Geometry: see drawing. Coordinates: mm, zero at the bounding-box minimum. A direction names the side the tool comes from. Round coordinates to 2 decimals unless told otherwise and drop trailing zeros. Order: outer loops, then holes, each group sorted by start corner. A loop starts at its lowest first (then second) coordinate and runs counter-clockwise, first axis right, second up. Notation, with made-up numbers: (58.25, 85.5) -> (112.25, 85.5) arc R19 cw to (112.25, 101.5) -> close; hole circle Ø1 at (69, -15.75). An arc over 180 degrees is marked (long way). Answer as CSV lines item,"result". Start each with the question number.
(1) Section query B-B (z = 15.3). Output: boundary loops of the cut face in (x, y).
(2) Line query: line 1 along Y through (x, z) = (11.5, 14.5); line 2 along X through (y, z) = (54, 21.5); line 3 along Y through (x, z) = (27.5, 7). Output: solid intervals per line, ascending. Write a range as from..to.
(3) Section query A-A (x = 15.3). Output: boundary loops of the cut face in (y, z), plus the area to 3 significant figures.
(4) Section query C-C (y = 44). Output: boundary loops of the cut face in (x, z).
(5) Section query D-D (x = 23). Output: boundary loops of the cut face in (y, z).
(6) Set-up query: the marked faces 1, 2 and 3. Return all of +Z, -Z, +X, -X, +Y, -Y with unobstructed straight access to the full face (end or side cutting, diameter ignored); none if empty.
(7) Contact query for flat-ended pins moving along their axis: P1, Ø5, axis at y = 37.5, z = 8.5, coming from the -X side; P2, Ø4, axis at x = 11, z = 10, coming from the +Y side; P3, Ø1, axis at x = 18, z = 6.5, coming from the -Y side. Output: stop coordinate, or through.
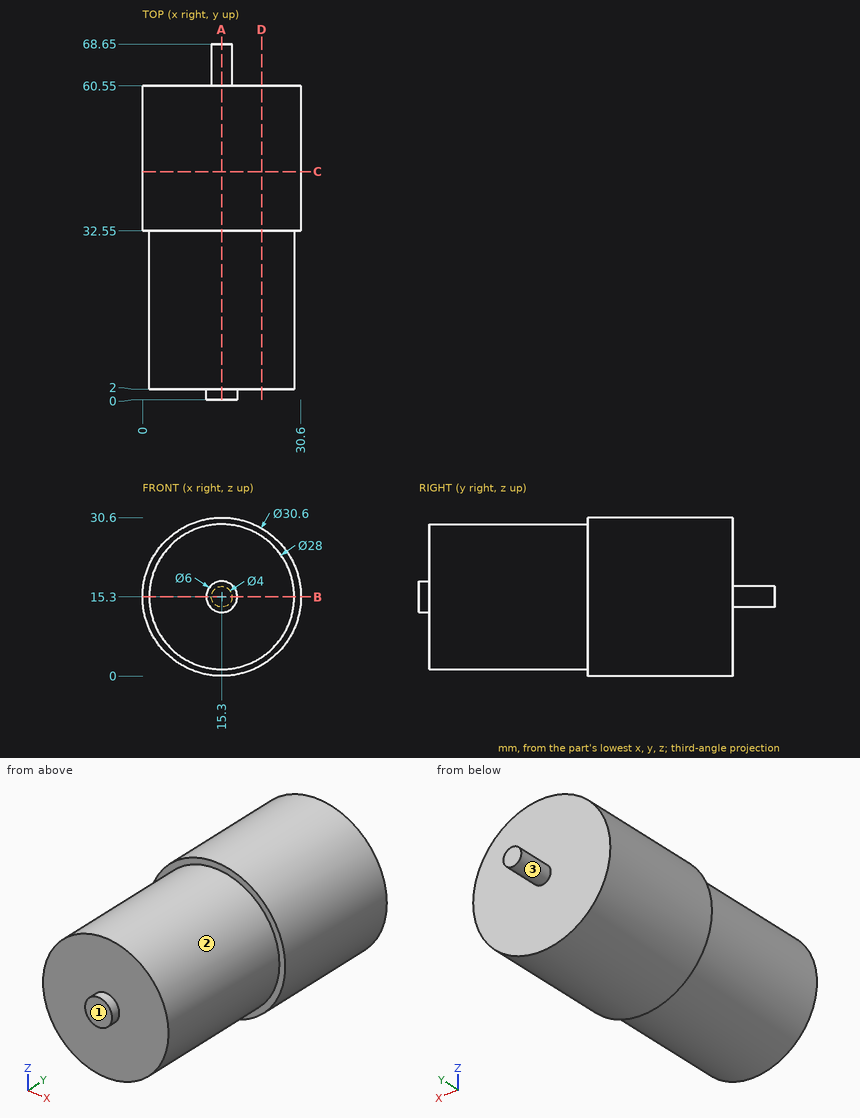
Answer block:
1,outline,"(0, 32.55) -> (1.3, 32.55) -> (1.3, 2) -> (12.3, 2) -> (12.3, 0) -> (18.3, 0) -> (18.3, 2) -> (29.3, 2) -> (29.3, 32.55) -> (30.6, 32.55) -> (30.6, 60.55) -> (17.3, 60.55) -> (17.3, 68.65) -> (13.3, 68.65) -> (13.3, 60.55) -> (0, 60.55) -> close"
2,line 1,"2..60.55"
2,line 2,"1.31..29.29"
2,line 3,"32.55..60.55"
3,outline,"(0, 12.3) -> (2, 12.3) -> (2, 1.3) -> (32.55, 1.3) -> (32.55, 0) -> (60.55, 0) -> (60.55, 13.3) -> (68.65, 13.3) -> (68.65, 17.3) -> (60.55, 17.3) -> (60.55, 30.6) -> (32.55, 30.6) -> (32.55, 29.3) -> (2, 29.3) -> (2, 18.3) -> (0, 18.3) -> close"
3,area,"1,760 mm2"
4,outline,"circle Ø30.6 at (15.3, 15.3)"
5,outline,"(2, 3.61) -> (32.55, 3.61) -> (32.55, 2.08) -> (60.55, 2.08) -> (60.55, 28.52) -> (32.55, 28.52) -> (32.55, 26.99) -> (2, 26.99) -> close"
6,face 1,"+Z, -Z, +X, -X, -Y"
6,face 2,"-Y"
6,face 3,"+Y"
7,P1,"x = 0.62"
7,P2,"y = 60.55"
7,P3,"y = 2"
